Could you check a few things on this model? Use its own coordinates, in mm. A direction names the side the tool comes from. Coordinates: 2 decimals unless noted, no trailing zeros. Loops run counter-clockwise (first coordinate to the right, second up) from the corner with the lowest first, then second, coordinate; pieces in that order, holes last. Notation, with made-up numbers: (5.25, 15.5) - (61.25, 15.5) arc R18 cw to (61.25, 46.5) - close; hole circle Ø8 at (39, 83.25). An arc over 180 degrees is marked (long way). Use CSV: the item, a comma, the result in double quotes.
from build123d import *

# Parameters (mm, degrees)
F0_W     = 622.3
F0_H     = 568.325
F0_R     = 4.7625
F0_R_2   = 2.54
F0_W_2   = 6.858
F0_H_2   = 6.858
F0_R_3   = 50.8
F1_DEPTH = 25.4
F2_T     = -2.54
F3_W     = 617.22
F3_H     = 22.86
F4_DEPTH = 563.245
F5_W     = 6.35
F5_H     = 3.175
F6_DEPTH = 568.326
F7_W     = 12.7
F7_H     = 107.95
F8_DEPTH = 2.54


with BuildPart() as f1:
    # F0 (on Front) → F1 (new body)
    with BuildSketch(Plane.XZ):
        with Locations((0, 284.1625)):
            Rectangle(F0_W, F0_H)
        with Locations((-292.1, 93.6625)):
            Circle(F0_R, mode=Mode.SUBTRACT)
        with Locations((-42.926, 241.2365)):
            Circle(F0_R_2, mode=Mode.SUBTRACT)
        with Locations((277.8125, 107.95)):
            Rectangle(F0_W_2, F0_H_2, mode=Mode.SUBTRACT)
        with Locations((42.926, 241.2365)):
            Circle(F0_R_2, mode=Mode.SUBTRACT)
        with Locations((277.8125, 158.75)):
            Rectangle(F0_W_2, F0_H_2, mode=Mode.SUBTRACT)
        with Locations((-42.926, 327.0885)):
            Circle(F0_R_2, mode=Mode.SUBTRACT)
        with Locations((-292.1, 474.6625)):
            Circle(F0_R, mode=Mode.SUBTRACT)
        with Locations((0, 284.1625)):
            Circle(F0_R_3, mode=Mode.SUBTRACT)
        with Locations((42.926, 327.0885)):
            Circle(F0_R_2, mode=Mode.SUBTRACT)
        with Locations((277.8125, 409.575)):
            Rectangle(F0_W_2, F0_H_2, mode=Mode.SUBTRACT)
        with Locations((277.8125, 460.375)):
            Rectangle(F0_W_2, F0_H_2, mode=Mode.SUBTRACT)
    extrude(amount=F1_DEPTH)

    # F2
    f2_openings = [f1.faces().sort_by_distance(p)[0] for p in [
        (302.722363, 0, 284.1625),
    ]]
    offset(amount=F2_T, openings=f2_openings, kind=Kind.INTERSECTION)

    # F3 (on face) → F4 (cut, through all)
    with BuildSketch(Plane.XY.offset(2.54)):
        with Locations((0, -11.43)):
            Rectangle(F3_W, F3_H)
    extrude(amount=F4_DEPTH, mode=Mode.SUBTRACT)

    # F5 (on face) → F6 (cut, through all)
    with BuildSketch(Plane.XY.offset(568.325)):
        with Locations((307.975, -1.5875)):
            Rectangle(F5_W, F5_H)
    extrude(amount=-F6_DEPTH, mode=Mode.SUBTRACT)

    # F7 (on face) → F8 (cut, through all)
    with BuildSketch(Plane.YZ.offset(311.15)):
        with Locations((-6.35, 434.975)):
            Rectangle(F7_W, F7_H)
        with Locations((-6.35, 133.35)):
            Rectangle(F7_W, F7_H)
    extrude(amount=-F8_DEPTH, mode=Mode.SUBTRACT)


solid = f1.part
(1) Suppose I cut it at D-D (x = 239). Write out the boundary of the cut face in (y, z) (3 decimals).
Computed:
outline,"(-25.4, 0) - (0, 0) - (0, 2.54) - (-22.86, 2.54) - (-22.86, 565.785) - (0, 565.785) - (0, 568.325) - (-25.4, 568.325) - close"
(2) Thinking about a two-plate mould opening in Z: for faces 3 (the face through (-4, -11, 565.785)), 4 (the face through (-4, -13, 568.325)), 5 (the face through (-4, -25.4, 225)), 6 (the face through (-308.61, -11, 280)), which applies, +Z half, -Z half, draft (parallel to the pull), parting line (faces both ways), or undercut?
Computed:
face 3,"undercut"
face 4,"+Z half"
face 5,"draft"
face 6,"undercut"
(3) Suppose I cut it at C-C (z = 206). Write out the boundary of the cut face in (x, y) (3 decimals).
Computed:
outline,"(-311.15, -25.4) - (311.15, -25.4) - (311.15, -3.175) - (308.61, -3.175) - (308.61, -22.86) - (-308.61, -22.86) - (-308.61, 0) - (-311.15, 0) - close"
(4) Please list where these lines run through material, in increasing order: line 1 (Z direction, x = -292.1, y = -24.35) (3 decimals); line 2 (X direction, y = -18.75, z = 529.5); line 3 (Z direction, x = 248, y = -1.75) (3 decimals).
Computed:
line 1,"z = 0 to 88.9, 98.425 to 469.9, 479.425 to 568.325"
line 2,"x = -311.15 to -308.61, 308.61 to 311.15"
line 3,"z = 0 to 2.54, 565.785 to 568.325"
(5) Will these pins go through, and if not, where does the flat tip stop? pin 1 (1.9 mm diameter, centred on x = 308, z = 513.5, fed in from +Y) (3 decimals); pin 2 (4.5 mm diameter, centred on x = 42.93, z = 241.24, fed in from -Y); pin 3 (0.8 mm diameter, centred on y = -2, z = 567.5, fed in from +X); pin 4 (1.5 mm diameter, centred on x = 104.5, z = 255.5, fed in from +Y).
Computed:
pin 1,"stops at y = -3.175"
pin 2,"passes through"
pin 3,"stops at x = 304.8"
pin 4,"stops at y = -22.86"
(6) Which directions (+Z, -Z, +X, -X, +Y, -Y) give clear straight access to the entire face, cutting with the end or side of a thin tool? Please do faces 1 (the face through (308.61, -15, 280)), 2 (the face through (23.441, -24.112, 239.094)).
Computed:
face 1,"+Y"
face 2,"+Y, -Y"
(7) Suppose I cut it at A-A (x = 0). Write out the boundary of the cut face in (y, z) (1 decimal).
Computed:
outline,"(-25.4, 0) - (0, 0) - (0, 2.5) - (-22.9, 2.5) - (-22.9, 233.4) - (-25.4, 233.4) - close; (-25.4, 335) - (-22.9, 335) - (-22.9, 565.8) - (0, 565.8) - (0, 568.3) - (-25.4, 568.3) - close"
(8) Suppose I cut it at B-B (y = -18). Write out the boundary of the cut face in (x, z) (3 decimals).
Computed:
outline,"(-311.15, 0) - (311.15, 0) - (311.15, 568.325) - (-311.15, 568.325) - close; hole (-308.61, 2.54) - (308.61, 2.54) - (308.61, 565.785) - (-308.61, 565.785) - close"
